```python
from build123d import *

# Parameters (mm, degrees)
V09_SPEAKER_BODY58P5X22P7X10_START = 23.65
SKETCH_2_W                         = 10
SKETCH_2_H                         = 58.5
V09_SPEAKER_BODY58P5X22P7X10_DEPTH = 22.7
V09_SPEAKER_LOWER_EAR_START        = 34.45
SKETCH_3_W                         = 1.5
SKETCH_3_H                         = 7.75
V09_SPEAKER_LOWER_EAR_DEPTH        = 11.9
V09_SPEAKER_UPPER_EAR_START        = 34.45
SKETCH_4_W                         = 1.5
SKETCH_4_H                         = 7.75
V09_SPEAKER_UPPER_EAR_DEPTH        = 11.9
SKETCH_5_R                         = 1.75
V09_SPEAKER_EAR_D3P5_PITCH66_DEPTH = 1.5


with BuildPart() as part:
    # 草图2 → V09_Speaker_body58p5x22p7x10 (new body)
    with BuildSketch(Plane.XY.offset(V09_SPEAKER_BODY58P5X22P7X10_START)):
        with Locations((150, -73)):
            Rectangle(SKETCH_2_W, SKETCH_2_H)
    extrude(amount=V09_SPEAKER_BODY58P5X22P7X10_DEPTH)

    # 草图3 → V09_Speaker_lower_ear (add)
    with BuildSketch(Plane.XY.offset(V09_SPEAKER_LOWER_EAR_START)):
        with Locations((154.25, -106.125)):
            Rectangle(SKETCH_3_W, SKETCH_3_H)
    extrude(amount=V09_SPEAKER_LOWER_EAR_DEPTH)

    # 草图4 → V09_Speaker_upper_ear (add)
    with BuildSketch(Plane.XY.offset(V09_SPEAKER_UPPER_EAR_START)):
        with Locations((154.25, -39.875)):
            Rectangle(SKETCH_4_W, SKETCH_4_H)
    extrude(amount=V09_SPEAKER_UPPER_EAR_DEPTH)

    # 草图5 → V09_Speaker_ear_D3p5_pitch66 (cut)
    with BuildSketch(Plane(origin=(155, 0, 0), x_dir=(0, 0, -1), z_dir=(1, 0, 0))):
        with Locations((-41.2, -106)):
            Circle(SKETCH_5_R)
        with Locations((-41.2, -40)):
            Circle(SKETCH_5_R)
    extrude(amount=-V09_SPEAKER_EAR_D3P5_PITCH66_DEPTH, mode=Mode.SUBTRACT)


solid = part.part
```
Source: CAD feature listing. Evaluate the final solid. Frame: model axes, mm. A direction names the side the tool comes from. Coordinates: 2 decimals unless noted, no trailing zeros. Loops run counter-clockwise (first coordinate to the right, second up) from the corner with the lowest first, then second, coordinate; pieces in that order, holes last. Notation, with made-up numbers: M -7.5,89 L 27.5,89 A18 cw 27.5,99 Z; hole C 27.5,21 d4. An arc over 180 degrees is marked long. Put each result on its own line as item: value. Start each with the question number.
1) Cut plane A-A on y = -40. Return the cut outline in (x, z), then the cut area to 3 significant figures.
2) Cut plane C-C on z = 26. Return the cut outline in (x, y), then the cut area to 3 significant figures.
3) Reachability of faces 1 (the face through (153.5, -40, 39)), 2 (the face through (154, -106, 34.45)), 3 (the face through (153.5, -106, 39)) from +Z, -Z, +X, -X, +Y, -Y: full face, straight path, thin tool, end or side. Return the list, or none.
4) Pull-direction query (Z, two-part tool) for faces 4 (the face through (150, -43.75, 35)), 5 (the face through (154.26, -106.67, 39.583)), 6 (the face through (150, -72, 46.35)); classes: pulls with the +Z half, pulls with the -Z half, needs draft (parallel to the pull), parting line crosses it, or undercut.
5) Cut plane B-B on z = 41.2. Return the cut outline in (x, y), then the cut area to 3 significant figures.
6) Cut plane D-D on x = 152.25. Return the cut outline in (y, z).
7) Ray query, L1, parallel to Y at x = 154.6, z = 41.2; L2, parallel to Z at x = 154.35, y = -106; L3, parallel to Y at x = 151, z = 42.25. Return the intervals inside material, ascending. Write a range as from..to.
8) Contact query for flat-ended pins moving along their axis: pin 1 Ø2 at (y, z) = (-40, 41.2) entering from -X; pin 2 Ø8.5 at (y, z) = (-38.5, 41.5) entering from -X; pin 3 Ø0.8 at (x, y) = (154.5, -39.5) entering from -Z. Output: stop coordinate, or through.
The answers:
1. outline: M 153.5,34.45 L 155,34.45 L 155,39.45 L 153.5,39.45 Z; M 153.5,42.95 L 155,42.95 L 155,46.35 L 153.5,46.35 Z
1. area: 12.6 mm²
2. outline: M 145,-102.25 L 155,-102.25 L 155,-43.75 L 145,-43.75 Z
2. area: 585 mm²
3. face 1: +Z, -Z, -X, +Y
3. face 2: -Z, +X, -X, -Y
3. face 3: +Z, -Z, -X, -Y
4. face 4: needs draft
4. face 5: undercut
4. face 6: pulls with the +Z half
5. outline: M 145,-102.25 L 153.5,-102.25 L 153.5,-104.25 L 155,-104.25 L 155,-41.75 L 153.5,-41.75 L 153.5,-43.75 L 145,-43.75 Z; M 153.5,-110 L 155,-110 L 155,-107.75 L 153.5,-107.75 Z; M 153.5,-38.25 L 155,-38.25 L 155,-36 L 153.5,-36 Z
5. area: 598 mm²
6. outline: M -102.25,23.65 L -43.75,23.65 L -43.75,46.35 L -102.25,46.35 Z
7. L1: y = -110..-107.75, -104.25..-41.75, -38.25..-36
7. L2: z = 34.45..39.45, 42.95..46.35
7. L3: y = -102.25..-43.75
8. pin 1: passes through
8. pin 2: stops at x = 153.5
8. pin 3: stops at z = 34.45
